from build123d import *

# Parameters (mm, degrees)
F0_W          = 38.1
F0_H          = 38.1
F0_W_2        = 32.004
F0_H_2        = 32.004
F1_DEPTH      = 228.6
F2_R          = 3.048
F3_R          = 6.35
F5_DEPTH      = 19.051
F5_DEPTH_BACK = 19.051
F7_DEPTH      = 19.051
F7_DEPTH_BACK = 19.051


with BuildPart() as f1:
    # F0 (on Top) → F1 (new body)
    with BuildSketch(Plane.XY):
        Rectangle(F0_W, F0_H)
        Rectangle(F0_W_2, F0_H_2, mode=Mode.SUBTRACT)
    extrude(amount=F1_DEPTH)

    # F2
    f2_edges = [f1.edges().sort_by_distance(p)[0] for p in [
        (16.002, 16.002, 114.3),
        (-16.002, 16.002, 114.3),
        (-16.002, -16.002, 114.3),
        (16.002, -16.002, 114.3),
    ]]
    fillet(f2_edges, radius=F2_R)

    # F3
    f3_edges = [f1.edges().sort_by_distance(p)[0] for p in [
        (-19.05, 19.05, 114.3),
        (-19.05, -19.05, 114.3),
        (19.05, -19.05, 114.3),
        (19.05, 19.05, 114.3),
    ]]
    fillet(f3_edges, radius=F3_R)

    # F4 (on Front) → F5 (cut, two sides)
    with BuildSketch(Plane.XZ) as f5_sk:
        Polygon((-19.05, 162.6088642316), (19.05, 228.6), (-19.05, 228.6), align=None)
    extrude(amount=-F5_DEPTH, mode=Mode.SUBTRACT)
    extrude(f5_sk.sketch, amount=F5_DEPTH_BACK, mode=Mode.SUBTRACT)

    # F6 (on Front) → F7 (cut, two sides)
    with BuildSketch(Plane.XZ) as f7_sk:
        Polygon((-19.05, 27.4963065702), (-19.05, 0), (28.575, 0), align=None)
    extrude(amount=-F7_DEPTH, mode=Mode.SUBTRACT)
    extrude(f7_sk.sketch, amount=F7_DEPTH_BACK, mode=Mode.SUBTRACT)


solid = f1.part
For this review, take the finished solid that the model builds, in its own axes (mm). A direction names the side the tool comes from. Round coordinates to 2 decimals unless told otherwise and drop trailing zeros. Write each loop counter-clockwise with the first axis right and the second up, starting at its lowest first coordinate (ties: lowest second). Pieces come first, ordered by that corner, then holes. Notation, with made-up numbers: (-33.75, 81.25) - (9.25, 81.25) arc R32 ccw to (9.25, 107.25) - close; hole circle Ø3 at (46.25, -22). An arc over 180 degrees is marked (long way). Use a Markdown table: item, result.
Q1. We need section D-D (z = 196). Give the boundary of the cut face in (x, y).
Derived:
| item | result |
|---|---|
| outline | (0.23, -19.05) - (12.7, -19.05) arc R6.35 ccw to (19.05, -12.7) - (19.05, 12.7) arc R6.35 ccw to (12.7, 19.05) - (0.23, 19.05) - (0.23, 16) - (12.95, 16) arc R3.05 cw to (16, 12.95) - (16, -12.95) arc R3.05 cw to (12.95, -16) - (0.23, -16) - close |
Q2. We need section B-B (y = -4). Give the boundary of the cut face in (x, z).
Derived:
| item | result |
|---|---|
| outline | (-19.05, 27.5) - (-16, 25.74) - (-16, 167.89) - (-19.05, 162.61) - close; (16, 7.26) - (19.05, 5.5) - (19.05, 228.6) - (16, 223.32) - close |
Q3. Machinability: for faces 1 (the flat face through (-16.002, 0, 96)), 2 (the flat face through (-19.05, 0, 94)), which of the approach directions +Z, -Z, +X, -X, +Y, -Y give a long, thin tool a straight path to every point of the face, cutting with its end or side? Answer none if there is none.
Derived:
| item | result |
|---|---|
| face 1 | +Z, -Z |
| face 2 | +Z, -Z, -X, +Y, -Y |
Q4. We need section A-A (z = 107.5). Give the boundary of the cut face in (x, y).
Derived:
| item | result |
|---|---|
| outline | (-19.05, -12.7) arc R6.35 ccw to (-12.7, -19.05) - (12.7, -19.05) arc R6.35 ccw to (19.05, -12.7) - (19.05, 12.7) arc R6.35 ccw to (12.7, 19.05) - (-12.7, 19.05) arc R6.35 ccw to (-19.05, 12.7) - close; hole (-16, -12.95) arc R3.05 ccw to (-12.95, -16) - (12.95, -16) arc R3.05 ccw to (16, -12.95) - (16, 12.95) arc R3.05 ccw to (12.95, 16) - (-12.95, 16) arc R3.05 ccw to (-16, 12.95) - close |
Q5. Clearance check with flat-ended pins moving along their axes: pin 1 (3 mm diameter, centred on x = 12.5, y = 13, fed in from +Z); pin 2 (4 mm diameter, centred on y = -15, z = 174, fed in from -X). State where each tip first meets the part, or that it passes through.
Derived:
| item | result |
|---|---|
| pin 1 | passes through |
| pin 2 | stops at x = -13.49 |
Q6. Wall thickness on line 1 along X through (y, z) = (4, 132); line 2 along X through (y, z) = (-13, 84.5): over which ranges is each line inside the solid? List them lowest first.
Derived:
| item | result |
|---|---|
| line 1 | x = -19.05 to -16, 16 to 19.05 |
| line 2 | x = -19.04 to -16, 16 to 19.04 |
Q7. We need section C-C (x = -6). Give the boundary of the cut face in (y, z).
Derived:
| item | result |
|---|---|
| outline | (-19.05, 19.96) - (-16, 19.96) - (-16, 185.21) - (-19.05, 185.21) - close; (16, 19.96) - (19.05, 19.96) - (19.05, 185.21) - (16, 185.21) - close |
